For this review, take the finished solid that the model builds, in its own axes (mm). A direction names the side the tool comes from. Give positions to 0.01 mm unless a question says otherwise; leave off trailing zeros. Order: outer loops, then holes, each group sorted by start corner. A loop starts at its lowest first (then second) coordinate and runs counter-clockwise, first axis right, second up. Notation, with made-up numbers: (87, 64.25) -> (126, 64.25) arc R13 cw to (126, 70.25) -> close; hole circle Ø6 at (1, 10.25). An arc over 180 degrees is marked (long way). Return JSON: item names as keys, results as strings. Group by question number.
1) Add section C-C (y = 0.25). Give the boundary of the cut face in (x, z), then the cut area to 3 significant figures.
2) The part is to be moulded in two halves that separate along Z. For faces 4 (the face through (-36.2, 1.5, 5.5)), 5 (the face through (10, -2.67, 3)), 6 (the face through (-8, 0, 0)), say which applies: released by +Z, released by -Z, zero draft, split by the parting line, or undercut.
3) Add section B-B (x = -22). Give the boundary of the cut face in (y, z).
4) Insertion check: P1, Ø5.5, axis at x = -37, z = 7, coming from the -Y side; P2, Ø2, axis at x = -16.5, z = 25, coming from the -Y side; P3, Ø2, axis at x = 10.5, y = -9, coming from the -Z side; P4, Ø4, axis at x = -35, z = 8, coming from the +Y side. Each pin has a flat end and moves straight along its axis. Give the tip position at first contact, or say it passes through.
5) Add section D-D (z = 7). State how many separate pieces and enclosed holes the cut face has, then the cut area to 3 significant figures.
6) For faces 1 (the face through (-37, 5, 15)), 2 (the face through (-35.82, 3.52, 4.35)), 3 (the face through (-10.75, -11, 14.79)), list the 3-axis set-ups (+Z, -Z, +X, -X, +Y, -Y) from which the entire face can be reached by the end or side of a thin tool; tool diameter is ignored.
7) To check wall thickness, follow line 1 along Y through (x, z) = (-22.5, 19.5); line 2 along Z through (x, y) = (8.3, 0); line 3 along X through (y, z) = (-3.5, 6). State the ranges of each line that lie inside material, in increasing order.
8) Add section A-A (z = 26). Give the boundary of the cut face in (x, y), then the cut area to 3 significant figures.
from build123d import *

# Parameters (mm, degrees)
SKETCH_W        = 53.671384
SKETCH_H        = 26
PAD_DEPTH       = 30
SKETCH001_W     = 15.2
SKETCH001_H     = 15.2
POCKET_DEPTH    = 30.001
SKETCH002_R     = 0.848528
SKETCH002_R_2   = 0.793369
POCKET001_DEPTH = 30.001
SKETCH003_W     = 2.8
SKETCH003_H     = 5.6
POCKET002_DEPTH = 6
SKETCH004_R     = 1.7
POCKET003_DEPTH = 6
SKETCH005_R     = 1.7
POCKET004_DEPTH = 17.001
POCKET005_DEPTH = 3
FILLET_R        = 2
FILLET001_R     = 2


with BuildPart() as part:
    # Sketch → Pad (new body)
    with BuildSketch(Plane.XY):
        with Locations((-14.164308, 0)):
            Rectangle(SKETCH_W, SKETCH_H)
    extrude(amount=PAD_DEPTH)

    # Sketch001 → Pocket (cut, through all)
    with BuildSketch(Plane(origin=(0, 0, 0), x_dir=(1, 0, 0), z_dir=(0, 0, -1))):
        Rectangle(SKETCH001_W, SKETCH001_H)
        with BuildLine():
            ThreePointArc((-30.947343, -1), (-13.000044, -0.055902), (-30.941113, 1))
            Line((-42, 1), (-30.941113, 1))
            Line((-42, -1), (-42, 1))
            Line((-30.947343, -1), (-42, -1))
        make_face()
        with BuildLine():
            ThreePointArc((-14, 8.944272), (-24.9794, 11.617839), (-33.325879, 4))
            Line((-43, 4), (-33.325879, 4))
            Line((-43, 4), (-43, 14))
            Line((-43, 14), (-6, 14))
            Line((-6, 14), (-14, 8.944272))
        make_face()
        with BuildLine():
            Line((-6, -14), (-43, -14))
            Line((-43, -14), (-43, -5))
            Line((-32.944272, -5), (-43, -5))
            ThreePointArc((-32.944272, -5), (-24.483382, -11.789328), (-14, -9))
            Line((-14, -9), (-6, -14))
        make_face()
    extrude(amount=-POCKET_DEPTH, mode=Mode.SUBTRACT)

    # Sketch002 → Pocket001 (cut, through all)
    with BuildSketch(Plane(origin=(0, 0, 0), x_dir=(1, 0, 0), z_dir=(0, 0, -1))):
        with Locations((7.6, -7.6)):
            Circle(SKETCH002_R)
        with Locations((-7.6, -7.6)):
            Circle(SKETCH002_R_2)
        with Locations((-7.6, 7.6)):
            Circle(SKETCH002_R)
        with Locations((7.6, 7.6)):
            Circle(SKETCH002_R)
    extrude(amount=-POCKET001_DEPTH, mode=Mode.SUBTRACT)

    # Sketch003 → Pocket002 (cut)
    with BuildSketch(Plane(origin=(0, 0, 0), x_dir=(1, 0, 0), z_dir=(0, 0, -1))):
        with Locations((10.009827, 8.414147)):
            Rectangle(SKETCH003_W, SKETCH003_H)
        with Locations((10.034181, -0.129832)):
            Rectangle(SKETCH003_W, SKETCH003_H)
    extrude(amount=-POCKET002_DEPTH, mode=Mode.SUBTRACT)

    # Sketch004 → Pocket003 (cut)
    with BuildSketch(Plane.YZ.offset(12.671384)):
        with Locations((0, 3)):
            Circle(SKETCH004_R)
        with Locations((-8.303802, 3)):
            Circle(SKETCH004_R)
    extrude(amount=-POCKET003_DEPTH, mode=Mode.SUBTRACT)

    # Sketch005 → Pocket004 (cut, through all)
    with BuildSketch(Plane.XZ.offset(4)):
        with Locations((-37, 7)):
            Circle(SKETCH005_R)
    extrude(amount=-POCKET004_DEPTH, mode=Mode.SUBTRACT)

    # Sketch006 → Pocket005 (cut)
    with BuildSketch(Plane(origin=(0, 5, 0), x_dir=(-1, 0, 0), z_dir=(0, 1, 0))):
        Polygon((39.692655, 8.990714), (36.622319, 10.327265), (33.929664, 8.336551), (34.307345, 5.009286), (37.377681, 3.672735), (40.070336, 5.663449), align=None)
    extrude(amount=-POCKET005_DEPTH, mode=Mode.SUBTRACT)

    # Fillet
    fillet_edges = [part.edges().sort_by_distance(p)[0] for p in [
        (2.54451, -13, 30),
        (12.671384, 0, 30),
        (2.535692, 13, 30),
        (-41, -2.5, 30),
        (-41, 3, 30),
    ]]
    fillet(fillet_edges, radius=FILLET_R)

    # Fillet001
    fillet001_edges = [part.edges().sort_by_distance(p)[0] for p in [
        (-41, 3, 0),
        (-41, -2.5, 0),
    ]]
    fillet(fillet001_edges, radius=FILLET001_R)


solid = part.part
Evaluation:
{
 "1": {"outline": "(-13, 0) -> (-7.6, 0) -> (-7.6, 30) -> (-13, 30) -> close; (7.6, 0) -> (8.63, 0) -> (8.63, 1.32) -> (7.6, 1.32) -> close; (7.6, 4.68) -> (8.63, 4.68) -> (8.63, 6) -> (11.43, 6) -> (11.43, 4.68) -> (12.67, 4.68) -> (12.67, 28) arc R2 ccw to (10.67, 30) -> (7.6, 30) -> close; (11.43, 0) -> (12.67, 0) -> (12.67, 1.32) -> (11.43, 1.32) -> close", "area": "289 mm^2"},
 "2": {"face 4": "undercut", "face 5": "zero draft", "face 6": "released by -Z"},
 "3": {"outline": "(-11.99, 0) -> (-8.97, 0) -> (-8.97, 30) -> (-11.99, 30) -> close; (9.03, 0) -> (12.05, 0) -> (12.05, 30) -> (9.03, 30) -> close"},
 "4": {"P1": "y = -4", "P2": "y = -11.12", "P3": "z = 0", "P4": "y = 5"},
 "5": {"separate pieces": "3", "enclosed holes": "1", "area": "594 mm^2"},
 "6": {"face 1": "+Z, -Z, -X, +Y", "face 2": "+Y", "face 3": "+Z, -Z, -Y"},
 "7": {"line 1": "-11.98 to -8.96, 9.01 to 12.04", "line 2": "0 to 1.3, 4.7 to 30", "line 3": "-41 to -38.37, -35.63 to -30.28, -13.72 to -7.6, 7.6 to 12.67"},
 "8": {"outline": "(-41, -4) -> (-33.33, -4) arc R12.02 ccw to (-14, -8.94) -> (-7.58, -13) -> (12.67, -13) -> (12.67, 13) -> (-7.6, 13) -> (-14, 9) arc R12.02 ccw to (-32.94, 5) -> (-41, 5) -> (-41, 1) -> (-30.95, 1) arc R9 cw (long way) to (-30.94, -1) -> (-41, -1) -> close; hole (-7.6, -6.75) arc R0.85 ccw (long way) to (-6.75, -7.6) -> (6.75, -7.6) arc R0.85 ccw (long way) to (7.6, -6.75) -> (7.6, 6.75) arc R0.85 ccw (long way) to (6.75, 7.6) -> (-6.81, 7.6) arc R0.79 ccw (long way) to (-7.6, 6.81) -> close", "area": "625 mm^2"}
}
